Autodesk Inventor part; units mm, degrees
ref_plane "YZ Plane" through (0, 0, 0) normal (1, 0, 0) x (0, 1, 0)
ref_plane "XZ Plane" through (0, 0, 0) normal (0, 1, 0) x (-1, 0, 0)
ref_plane "XY Plane" through (0, 0, 0) normal (0, 0, 1) x (1, 0, 0)
sketch "Sketch1" plane through (0, 0, 0) normal (1, 0, 0) x (0, 1, 0)
  line L0 (0, 0) -> (0, 660.4)
  line L1 (0, 330.2) -> (453.6585, 330.2) construction
  line L2 (453.6585, 431.8) -> (453.6585, 330.2)
  line L3 (453.6585, 330.2) -> (453.6585, 228.6)
  line L4 (453.6585, 431.8) -> (0, 660.4)
  line L5 (453.6585, 228.6) -> (0, 0)
  dimension "d0" = 660.4
  dimension "d4" = 203.2
  dimension "d29" = 228.6
  dimension "d31" = 508
  dimension "d32" = 453.6585
extrude "Extrusion1" add sketch "Sketch1" along normal blind 3.175
properties part number "Polycarb Side1 Pannel" material "Polycarbonate, Clear"
Geometry check sheet. Reference: the model listing, model coordinates, mm. Coordinates: 2 decimals unless noted, no trailing zeros. Write each loop counter-clockwise with the first axis right and the second up, starting at its lowest first coordinate (ties: lowest second). Pieces come first, ordered by that corner, then holes. Notation, with made-up numbers: M 56,21 L 92,21 A14 cw 92,32 Z; hole C 87,78.25 d9. An arc over 180 degrees is marked long. One line per item, written item: value. Start each with the question number.
(1) Depth check by flat-ended pin: pin 1 (1.5 mm diameter, centred on x = 1, z = 488, fed in from +Y); pin 2 (1.5 mm diameter, centred on x = 2, y = 66.5, fed in from +Z). Enter the tip coordinate at first touch or a pass-through.
(2) Scan lines: line 1 along Z through (x, y) = (2.75, 320); line 2 along Z through (x, y) = (0.55, 58.5); line 3 along Y through (x, z) = (2.2, 141.5). Record each from-to range of solid material in increasing order. Write a range as [from, to].
(3) Sectioned sample at A-A, the plane x = 2.6. Enter the section's corners in (y, z).
(4) Sectioned sample at B-B, the plane y = 289. Enter the section's corners in (x, z) (3 decimals).
Filled sheet:
1. pin 1: y = 343.62
1. pin 2: z = 627.27
2. line 1: [161.25, 499.15]
2. line 2: [29.48, 630.92]
2. line 3: [0, 280.81]
3. outline: M 0,0 L 453.66,228.6 L 453.66,431.8 L 0,660.4 Z
4. outline: M 0,145.628 L 3.175,145.628 L 3.175,514.772 L 0,514.772 Z
